Geometry: see drawing. Coordinates: mm, zero at the bounding-box minimum. A direction names the side the tool comes from. Round coordinates to 2 decimals unless told otherwise and drop trailing zeros. Write each loop counter-clockwise with the first axis right and the second up, starting at its lowest first coordinate (ties: lowest second). Pieces come first, ordered by that corner, then holes. Notation, with made-up numbers: (-30, -20) -> (3, -20) arc R32 cw to (3, 8) -> close; hole circle Ø3 at (20, 43). An arc over 180 degrees is marked (long way). Write item = value, one per line.
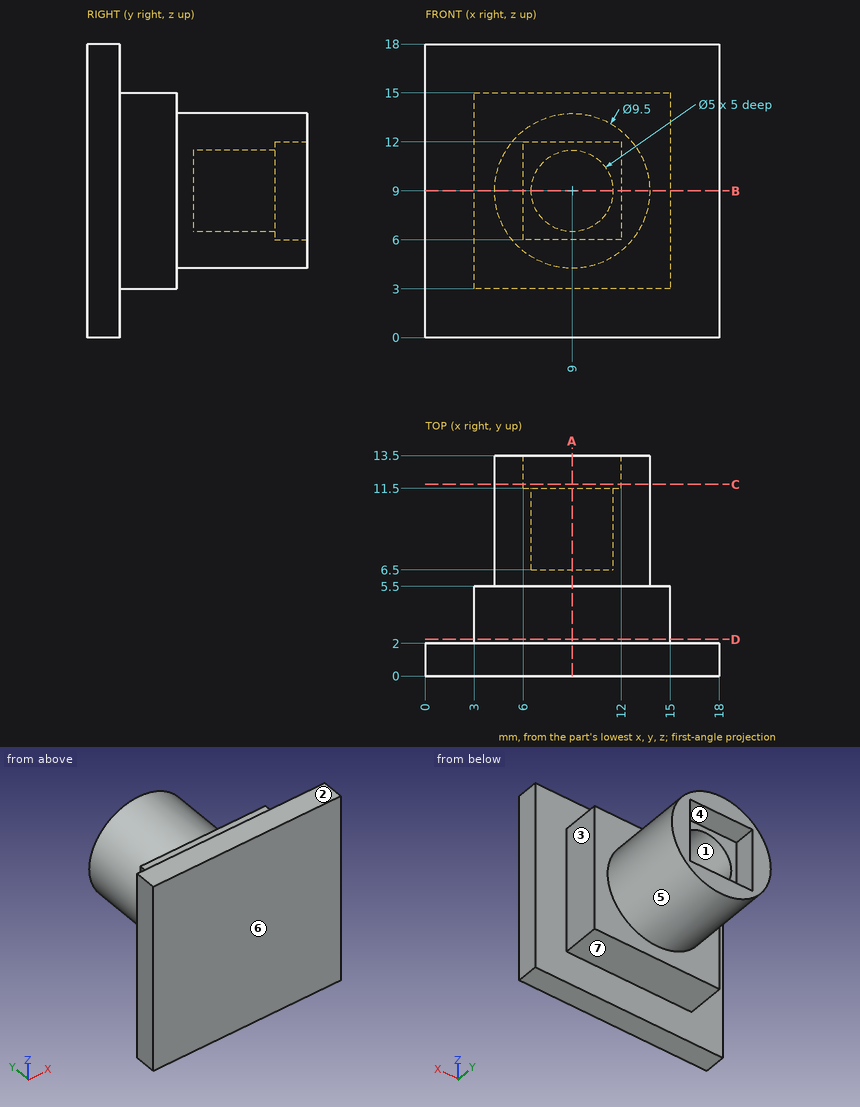
1) Cut plane C-C (y = 11.75). Return the cut outline in (x, z), and give its area (3 significant figures).
Solutions:
outline = circle Ø9.5 at (9, 9); hole (6, 6) -> (12, 6) -> (12, 12) -> (6, 12) -> close
area = 34.9 mm^2
2) Access query for the marked faces 5, 6 and 7. Directions: +Z, -Z, +X, -X, +Y, -Y. A direction counts if a zero-diameter tool reaches every point of the face in a straight line with its end or side. Return the directions, or none.
Solutions:
face_5 = +Y
face_6 = +Z, -Z, +X, -X, -Y
face_7 = -Z, +X, -X, +Y
3) First-contact query: P1, Ø5, axis at x = 11.5, y = 4, coming from the +Z side; P2, Ø1.8, axis at x = 11.5, y = 3.5, coming from the -Z side; P3, Ø2, axis at y = 12, z = 8, coming from the -X side; P4, Ø0.6, axis at x = 9.5, y = 12, coming from the -Z side. Flat tips, straight axial feed; report the tip coordinate or a pass-through.
Solutions:
P1 = 18
P2 = 3
P3 = 4.25
P4 = 4.25
4) Cut plane B-B (z = 9). Return the cut outline in (x, y), and give its area (3 significant figures).
Solutions:
outline = (0, 0) -> (18, 0) -> (18, 2) -> (15, 2) -> (15, 5.5) -> (13.75, 5.5) -> (13.75, 13.5) -> (12, 13.5) -> (12, 11.5) -> (11.5, 11.5) -> (11.5, 6.5) -> (6.5, 6.5) -> (6.5, 11.5) -> (6, 11.5) -> (6, 13.5) -> (4.25, 13.5) -> (4.25, 5.5) -> (3, 5.5) -> (3, 2) -> (0, 2) -> close
area = 117 mm^2
5) Line query: L1, parallel to Z at x = 9, y = 10; L2, parallel to Y at x = 13, z = 14.5; L3, parallel to Y at x = 10.75, z = 16.25. Output: solid intervals per line, ascending. Write a range as from..to.
Solutions:
L1 = 4.25..6.5, 11.5..13.75
L2 = 0..5.5
L3 = 0..2
6) Cut plane A-A (x = 9). Return the cut outline in (y, z).
Solutions:
outline = (0, 0) -> (2, 0) -> (2, 3) -> (5.5, 3) -> (5.5, 4.25) -> (13.5, 4.25) -> (13.5, 6) -> (11.5, 6) -> (11.5, 6.5) -> (6.5, 6.5) -> (6.5, 11.5) -> (11.5, 11.5) -> (11.5, 12) -> (13.5, 12) -> (13.5, 13.75) -> (5.5, 13.75) -> (5.5, 15) -> (2, 15) -> (2, 18) -> (0, 18) -> close
7) Draft query along X for the marked faces 1, 2, 3 and 4. Return one class per face: +X half, -X half, draft (parallel to the pull), parting line (faces both ways), or undercut.
Solutions:
face_1 = undercut
face_2 = draft
face_3 = +X half
face_4 = undercut
8) Cut plane D-D (y = 2.25). Return the cut outline in (x, z), and give its area (3 significant figures).
Solutions:
outline = (3, 3) -> (15, 3) -> (15, 15) -> (3, 15) -> close
area = 144 mm^2
